The figure shows three views and two pictorial views of one solid part (mm, origin at its lowest corner). Answer the questions. A direction names the side the tool comes from. Coordinates: 2 decimals unless noted, no trailing zeros. Loops run counter-clockwise (first coordinate to the right, second up) from the corner with the lowest first, then second, coordinate; pieces in that order, holes last. Notation, with made-up numbers: (31, 76) - (60, 76) arc R28 cw to (60, 104) - close; hole circle Ø9 at (-26, 57.5). An arc over 180 degrees is marked (long way). One line per question, with ' | ' between items.
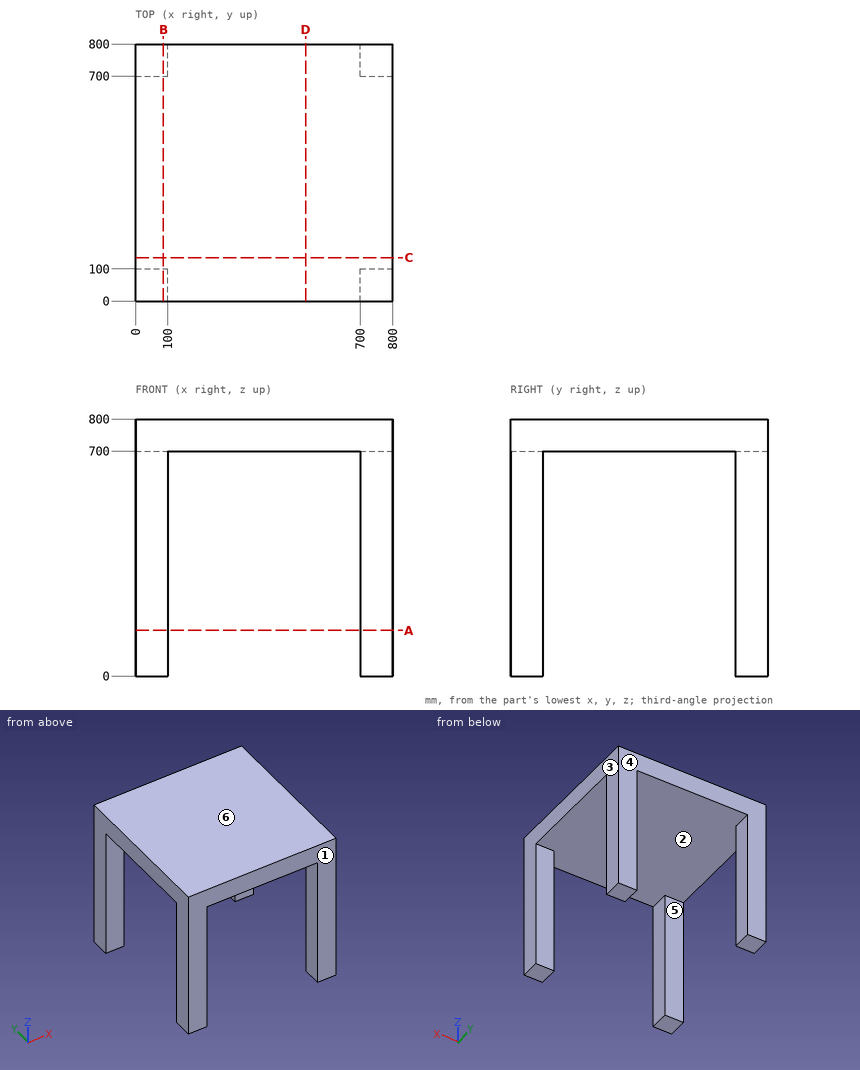
Item 1: This flat-tipped pin is pushed along its axis until it touches: pin 1 Ø5 at (x, y) = (686, 658.5) entering from -Z. Where does it stop, or does it pass through?
Taken from the geometry:
pin 1: stops at z = 700
Item 2: Find the intervals of material crossed by line 1 (X direction, y = 86, z = 422); line 2 (Z direction, x = 476.5, y = 579), in increasing order. Write a range as [from, to].
Taken from the geometry:
line 1: x = [0, 100], [700, 800] | line 2: z = [700, 800]
Item 3: Find section C-C, the plane y = 135. Write down the section's boundary in (x, z).
Taken from the geometry:
outline: (0, 700) - (800, 700) - (800, 800) - (0, 800) - close
Item 4: Find section B-B, the plane x = 87. Write down the section's boundary in (y, z).
Taken from the geometry:
outline: (0, 0) - (100, 0) - (100, 700) - (700, 700) - (700, 0) - (800, 0) - (800, 800) - (0, 800) - close
Item 5: Find section A-A, the plane z = 142. Write down the section's boundary in (x, y).
Taken from the geometry:
outline: (0, 0) - (100, 0) - (100, 100) - (0, 100) - close; (0, 700) - (100, 700) - (100, 800) - (0, 800) - close; (700, 0) - (800, 0) - (800, 100) - (700, 100) - close; (700, 700) - (800, 700) - (800, 800) - (700, 800) - close
Item 6: The mould has two halves that part along Y. Classify the marked faces 1, 2, 3 and 4: pulls with the +Y half, pulls with the -Y half, needs draft (parallel to the pull), parting line crosses it, or undercut.
Taken from the geometry:
face 1: pulls with the -Y half | face 2: undercut | face 3: needs draft | face 4: pulls with the +Y half
Item 7: Which of the six approach directions +Z, -Z, +X, -X, +Y, -Y give full straight-line access (tool end or side, diameter ignored) to the marked faces 5 and 6?
Taken from the geometry:
face 5: -Z, +X, -X | face 6: +Z, +X, -X, +Y, -Y
